from build123d import *

# Parameters (mm, degrees)
SKETCH1_R                        = 103
BASE_DISC_DEPTH                  = 1.5
SKETCH3_R                        = 3
CUT_EXTRUDE1_DEPTH               = 146.671719973
SKETCH4_RX                       = 28
SKETCH4_RY                       = 16
CUT_EXTRUDE2_DEPTH               = 146.671719973
SKETCH2_R                        = 7.5
CUT_EXTRUDE3_DEPTH               = 146.671720116
CIRPATTERN3_COUNT                = 4
CIRPATTERN4_COUNT                = 4
SKETCH5_R                        = 1.4
CUT_EXTRUDE4_DEPTH               = 146.671720116
SKETCH6_R                        = 7.51
SKETCH6_R_2                      = 7
CENTRE_BORE_CORRECTION_D14_DEPTH = 1.5


with BuildPart() as part:
    # Sketch1 → Base Disc (new body)
    with BuildSketch(Plane.XY):
        Circle(SKETCH1_R)
    extrude(amount=BASE_DISC_DEPTH)

    # Sketch3 → Cut-Extrude1 (cut, through all)
    with BuildSketch(Plane(origin=(0, 0, 0), x_dir=(-1, 0, 0), z_dir=(0, 0, -1))):
        with Locations((95, 0)):
            Circle(SKETCH3_R)
    cut_extrude1 = extrude(amount=-CUT_EXTRUDE1_DEPTH, mode=Mode.SUBTRACT)

    # Sketch4 → Cut-Extrude2 (cut, through all)
    with BuildSketch(Plane(origin=(0, 0, 0), x_dir=(-1, 0, 0), z_dir=(0, 0, -1))):
        with Locations(Location((38.890872965, 38.890872965), (0, 0, 135))):
            Ellipse(SKETCH4_RX, SKETCH4_RY)
    cut_extrude2 = extrude(amount=-CUT_EXTRUDE2_DEPTH, mode=Mode.SUBTRACT)

    # Sketch2 → Cut-Extrude3 (cut, through all)
    with BuildSketch(Plane(origin=(0, 0, 0), x_dir=(-1, 0, 0), z_dir=(0, 0, -1))):
        Circle(SKETCH2_R)
    extrude(amount=-CUT_EXTRUDE3_DEPTH, mode=Mode.SUBTRACT)

    # CirPattern3: Cut-Extrude1 ×4 about axis
    cirpattern3_axis = Axis((0, 0, 0), (0, 0, 1))
    for i in range(1, CIRPATTERN3_COUNT):
        add(cut_extrude1.rotate(cirpattern3_axis, i * 360 / CIRPATTERN3_COUNT), mode=Mode.SUBTRACT)

    # CirPattern4: Cut-Extrude2 ×4 about axis
    cirpattern4_axis = Axis((0, 0, 0), (0, 0, -1))
    for i in range(1, CIRPATTERN4_COUNT):
        add(cut_extrude2.rotate(cirpattern4_axis, i * 360 / CIRPATTERN4_COUNT), mode=Mode.SUBTRACT)

    # Sketch5 → Cut-Extrude4 (cut, through all)
    with BuildSketch(Plane.XY):
        with Locations((-7.778174593, -7.778174593)):
            Circle(SKETCH5_R)
        with Locations((-7.778174593, 7.778174593)):
            Circle(SKETCH5_R)
        with Locations((7.778174593, 7.778174593)):
            Circle(SKETCH5_R)
        with Locations((7.778174593, -7.778174593)):
            Circle(SKETCH5_R)
    extrude(amount=CUT_EXTRUDE4_DEPTH, mode=Mode.SUBTRACT)

    # Sketch6 → Centre_Bore_Correction_D14 (add)
    with BuildSketch(Plane.XY):
        Circle(SKETCH6_R)
        Circle(SKETCH6_R_2, mode=Mode.SUBTRACT)
    extrude(amount=CENTRE_BORE_CORRECTION_D14_DEPTH)


solid = part.part
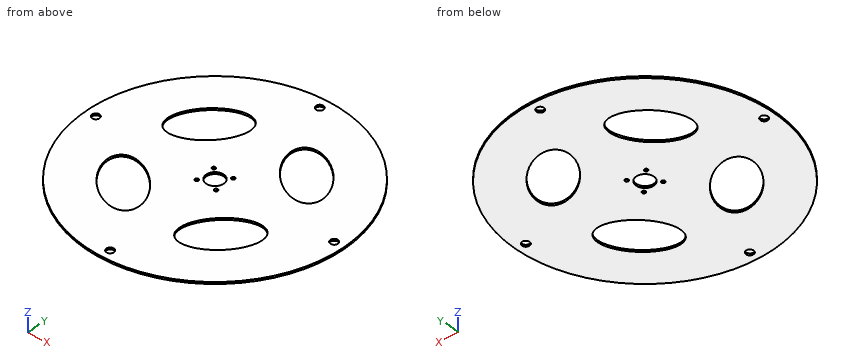
Build history of the part. All positions in model axes, mm. Round coordinates to 2 decimals unless told otherwise and drop trailing zeros. Write each loop counter-clockwise with the first axis right and the second up, starting at its lowest first coordinate (ties: lowest second). Pieces come first, ordered by that corner, then holes. Notation, with made-up numbers: (47.25, 15.5) -> (99.25, 15.5) arc R32 ccw to (99.25, 46.5) -> close; hole circle Ø6 at (39.25, 59.5). An arc over 180 degrees is marked (long way). Write item = value, one per line.
(1) Band-saw the part on D-D (y = -50.5). State how many separate pieces and enclosed holes the cut face has, then the cut area to 3 significant figures.
Answer:
separate_pieces = 3
enclosed_holes = 0
area = 168 mm2
(2) Probe L1, parallel to Y at x = 49, z = 0.5; L2, parallel to Y at x = -56, z = 0.4; L3, parallel to X at y = -20.5, z = 0.6. List the from-to ranges inside material, lowest first.
Answer:
L1 = -90.6 to -51.37, -16.15 to 16.15, 51.37 to 90.6
L2 = -86.45 to -43.19, -17.22 to 17.22, 43.19 to 86.45
L3 = -100.94 to -59.84, -36.61 to 36.61, 59.84 to 100.94
(3) Band-saw the part on B-B (x = 0). Give the cut face in (y, z), then the cut area to 3 significant figures.
Answer:
outline = (-103, 0) -> (-98, 0) -> (-98, 1.5) -> (-103, 1.5) -> close; (-92, 0) -> (-7, 0) -> (-7, 1.5) -> (-92, 1.5) -> close; (7, 0) -> (92, 0) -> (92, 1.5) -> (7, 1.5) -> close; (98, 0) -> (103, 0) -> (103, 1.5) -> (98, 1.5) -> close
area = 270 mm2
(4) Flat gauge pins, fed straight in: pin 1 (8 mm diameter, centred on x = 32, y = -61, fed in from +Z); pin 2 (5 mm diameter, centred on x = 0, y = -95, fed in from +Z). Where does each tip first touch, or does it go through?
Answer:
pin_1 = 1.5
pin_2 = through
(5) Band-saw the part on A-A (x = 95). Give the cut face in (y, z).
Answer:
outline = (-39.8, 0) -> (-3, 0) -> (-3, 1.5) -> (-39.8, 1.5) -> close; (3, 0) -> (39.8, 0) -> (39.8, 1.5) -> (3, 1.5) -> close
